Study the drawing (mm; zero at the part's minimum x, y, z) and answer. Round coordinates to 2 decimals unless told otherwise and drop trailing zeros. Write each loop counter-clockwise with the first axis right and the second up, starting at its lowest first coordinate (ties: lowest second). Pieces come first, ordered by that corner, then holes.
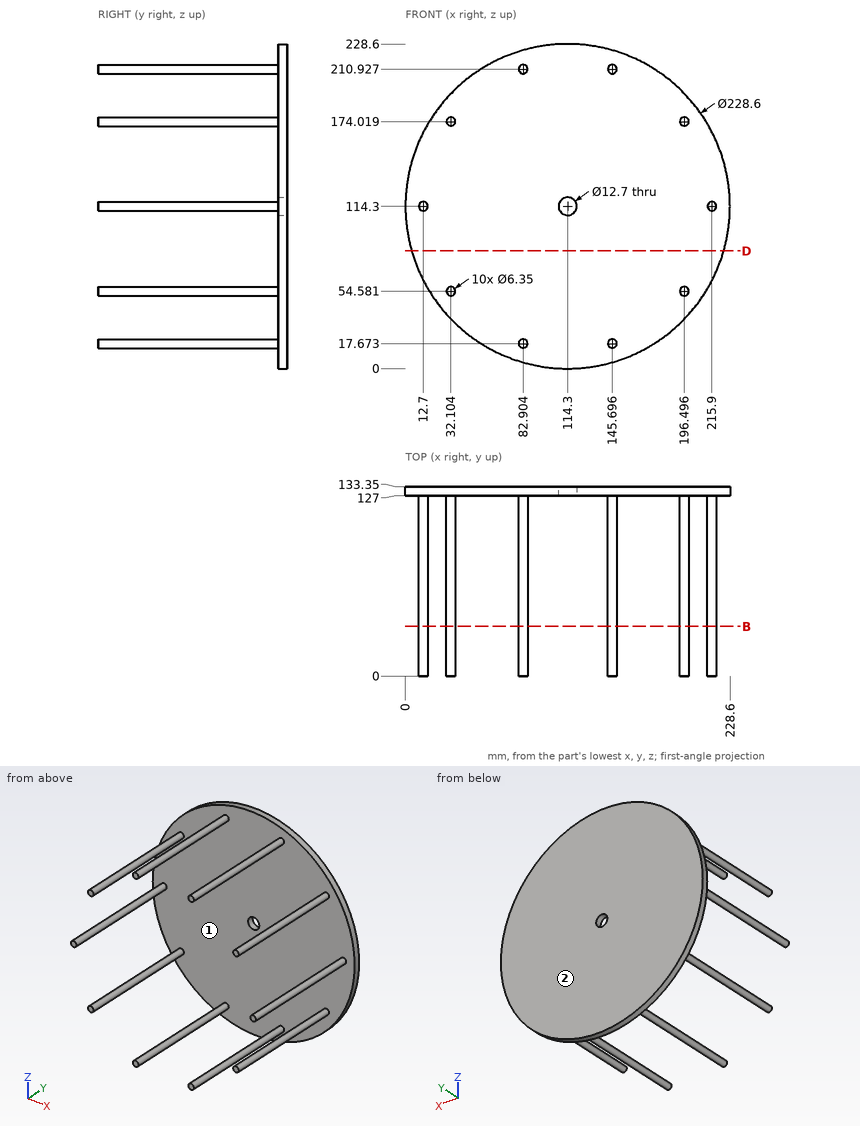
1. For a pull along Y with two mould halves and no side action, classify the marked faces 1 and 2 as released by +Y, released by -Y, zero draft, split by the parting line, or undercut.
Geometry says:
face 1: released by -Y
face 2: released by +Y
2. Section D-D on z = 83 is taken. Determine the outline of the cut face in (x, y), plus the area to 3 significant figures.
Geometry says:
outline: (4.37, 127) - (224.23, 127) - (224.23, 133.35) - (4.37, 133.35) - close
area: 1,400 mm2
3. Given pin 1 (5 mm diameter, centred on x = 79.5, y = 72.5, fed in from -Z); pin 2 (12 mm diameter, centred on x = 171, z = 161, fed in from -Y); pin 3 (5 mm diameter, centred on y = 40, z = 204.5, fed in from -X); pin 4 (12 mm diameter, centred on x = 137.5, y = 31.5, fed in from -Z), each flat-ended and moving along its own axis, determine where each tip first touches the part or whether it passes through.
Geometry says:
pin 1: stops at z = 14.63
pin 2: stops at y = 127
pin 3: passes through
pin 4: stops at z = 15.38
4. Straight lines are drawn through the part: line 1 along X through (y, z) = (90.5, 211); line 2 along Z through (x, y) = (114.3, 130.25); line 3 along Y through (x, z) = (51, 90). For each, find the intervals that lie inside material, in ascending order.
Geometry says:
line 1: x = 79.73 to 86.08, 142.52 to 148.87
line 2: z = 0 to 107.95, 120.65 to 228.6
line 3: y = 127 to 133.35
5. Section B-B on y = 35 is taken. Give the number of separate pieces and of enclosed holes in the cut face, plus the area to 3 significant figures.
Geometry says:
separate pieces: 10
enclosed holes: 0
area: 317 mm2
